from build123d import *

# Parameters (mm, degrees)
SKETCH1_W           = 101.6
SKETCH1_H           = 76.835
BOSS_EXTRUDE1_DEPTH = 1.5875
SKETCH2_R           = 4.7625
CUT_EXTRUDE1_DEPTH  = 2.5875


with BuildPart() as part:
    # Sketch1 → Boss-Extrude1 (new body)
    with BuildSketch(Plane(origin=(0, 0, 0), x_dir=(0, 0, -1), z_dir=(1, 0, 0))):
        Rectangle(SKETCH1_W, SKETCH1_H)
    extrude(amount=BOSS_EXTRUDE1_DEPTH)

    # Sketch2 → Cut-Extrude1 (cut, through all)
    with BuildSketch(Plane(origin=(1.5875, 0, 0), x_dir=(0, 0, -1), z_dir=(1, 0, 0))):
        with Locations((-38.1, -25.7175)):
            Circle(SKETCH2_R)
        with Locations((-12.7, -25.7175)):
            Circle(SKETCH2_R)
        with Locations((12.7, -25.7175)):
            Circle(SKETCH2_R)
        with Locations((38.1, -25.7175)):
            Circle(SKETCH2_R)
        with BuildLine():
            Line((-36.195, -2.2987), (-23.495, -2.2987))
            ThreePointArc((-23.495, -2.2987), (-20.955, -4.8387), (-23.495, -7.3787))
            Line((-23.495, -7.3787), (-36.195, -7.3787))
            ThreePointArc((-36.195, -7.3787), (-38.735, -4.8387), (-36.195, -2.2987))
        make_face()
        with BuildLine():
            Line((27.305, -2.2987), (40.005, -2.2987))
            ThreePointArc((40.005, -2.2987), (42.545, -4.8387), (40.005, -7.3787))
            Line((40.005, -7.3787), (27.305, -7.3787))
            ThreePointArc((27.305, -7.3787), (24.765, -4.8387), (27.305, -2.2987))
        make_face()
        with BuildLine():
            Line((27.305, 29.4513), (40.005, 29.4513))
            ThreePointArc((40.005, 29.4513), (42.545, 26.9113), (40.005, 24.3713))
            Line((40.005, 24.3713), (27.305, 24.3713))
            ThreePointArc((27.305, 24.3713), (24.765, 26.9113), (27.305, 29.4513))
        make_face()
        with BuildLine():
            Line((-36.195, 29.4513), (-23.495, 29.4513))
            ThreePointArc((-23.495, 29.4513), (-20.955, 26.9113), (-23.495, 24.3713))
            Line((-23.495, 24.3713), (-36.195, 24.3713))
            ThreePointArc((-36.195, 24.3713), (-38.735, 26.9113), (-36.195, 29.4513))
        make_face()
        with BuildLine():
            Line((-4.445, 26.9113), (8.255, 26.9113))
            ThreePointArc((8.255, 26.9113), (24.13, 11.0363), (8.255, -4.8387))
            Line((8.255, -4.8387), (-4.445, -4.8387))
            ThreePointArc((-4.445, -4.8387), (-20.32, 11.0363), (-4.445, 26.9113))
        make_face()
    extrude(amount=-CUT_EXTRUDE1_DEPTH, mode=Mode.SUBTRACT)


solid = part.part
Geometry check sheet. Reference: the model listing, model coordinates, mm. A direction names the side the tool comes from. Give positions to 0.01 mm unless a question says otherwise; leave off trailing zeros. Loops run counter-clockwise (first coordinate to the right, second up) from the corner with the lowest first, then second, coordinate; pieces in that order, holes last. Notation, with made-up numbers: (46.25, -15) -> (97.25, -15) arc R11 cw to (97.25, 0) -> close; hole circle Ø10 at (67.5, 68.5). An arc over 180 degrees is marked (long way). Answer in a Markdown table with one row per item. Add a question column.
1) Set-up check for faces 1 (the face through (1.588, -8, 1)), 2 (the face through (0.805, -4.895, -24.766)): record each of +Z, -Z, +X, -X, +Y, -Y from which the full face is reachable in a straight line by a thin tool's end or side.
2) Draft check along Y on faces 3 (the face through (0.805, 26.855, 38.734)), 4 (the face through (0, -8, 1)). Enter one of: pulls with the +Y half, pulls with the -Y half, needs draft (parallel to the pull), parting line crosses it, or undercut.
3) Cross-section at B-B on y = 20.5. Record the boundary of the cut face in (x, z).
4) Cross-section at D-D on z = -19.5. Record the boundary of the cut face in (x, y), and give its area (3 significant figures).
5) Material ranges on probe 1 along Z at (x, y) = (0.1, -25.5); probe 2 along Y at (x, z) = (1.1, 26); probe 3 along Y at (x, z) = (0.95, -38.1) (1 decimal), recorded low to high. Write a range as from..to.
6) Cross-section at A-A on z = 32. Record the boundary of the cut face in (x, y), and give its area (3 significant figures).
7) Cross-section at C-C on y = -27. Record the boundary of the cut face in (x, z).
8) Gauge pin test, flat end, axial feed: P1, Ø5.5, axis at y = -25.72, z = -38.1, coming from the +X side. Record the tip position at first contact, or that the pin passes through.
Outcome:
| question | item | result |
|---|---|---|
| 1 | face 1 | +Z, -Z, +X, +Y, -Y |
| 1 | face 2 | +X, -X |
| 2 | face 3 | undercut |
| 2 | face 4 | needs draft |
| 3 | outline | (0, -50.8) -> (1.59, -50.8) -> (1.59, -21) -> (0, -21) -> close; (0, 17.19) -> (1.59, 17.19) -> (1.59, 50.8) -> (0, 50.8) -> close |
| 4 | outline | (0, -38.42) -> (1.59, -38.42) -> (1.59, -0.17) -> (0, -0.17) -> close; (0, 22.24) -> (1.59, 22.24) -> (1.59, 38.42) -> (0, 38.42) -> close |
| 4 | area | 86.4 mm^2 |
| 5 | probe 1 | z = -50.8..-42.86, -33.34..-17.46, -7.94..7.94, 17.46..33.34, 42.86..50.8 |
| 5 | probe 2 | y = -38.42..-7.38, -2.3..24.37, 29.45..38.42 |
| 5 | probe 3 | y = -38.4..-30.5, -21..-7.4, -2.3..24.4, 29.5..38.4 |
| 6 | outline | (0, -38.42) -> (1.59, -38.42) -> (1.59, -7.38) -> (0, -7.38) -> close; (0, -2.3) -> (1.59, -2.3) -> (1.59, 24.37) -> (0, 24.37) -> close; (0, 29.45) -> (1.59, 29.45) -> (1.59, 38.42) -> (0, 38.42) -> close |
| 6 | area | 106 mm^2 |
| 7 | outline | (0, -50.8) -> (1.59, -50.8) -> (1.59, -42.69) -> (0, -42.69) -> close; (0, -33.51) -> (1.59, -33.51) -> (1.59, -17.29) -> (0, -17.29) -> close; (0, -8.11) -> (1.59, -8.11) -> (1.59, 8.11) -> (0, 8.11) -> close; (0, 17.29) -> (1.59, 17.29) -> (1.59, 33.51) -> (0, 33.51) -> close; (0, 42.69) -> (1.59, 42.69) -> (1.59, 50.8) -> (0, 50.8) -> close |
| 8 | P1 | passes through |
